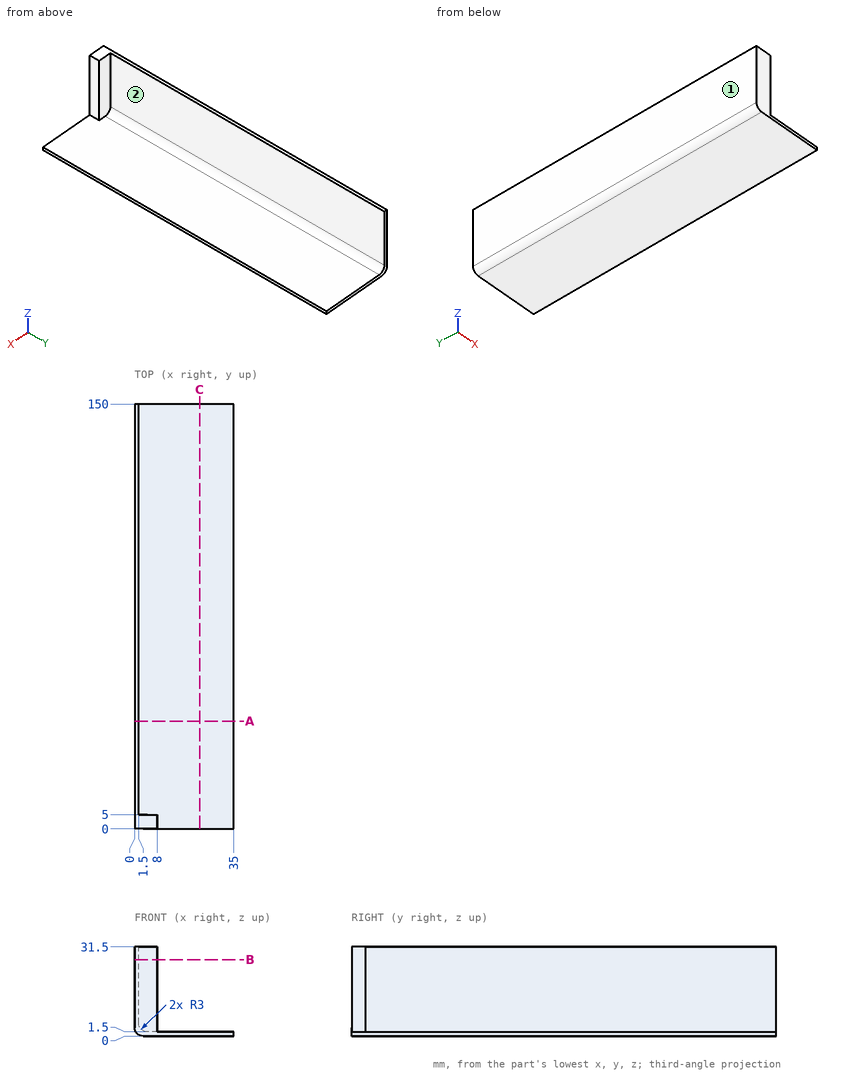
Answer from the drawing. Dimensions are ordinates in mm from the lowest x, y and z of the part. A direction names the side the tool comes from. Coordinates: 2 decimals unless noted, no trailing zeros. Order: outer loops, then holes, each group sorted by start corner. A loop starts at its lowest first (then second) coordinate and runs counter-clockwise, first axis right, second up. Notation, with made-up numbers: M 85,88 L 114,88 A9 ccw 114,99 Z; hole C 62.5,10.5 d6. An arc over 180 degrees is marked long. Put each result on its own line as item: value. Start each with the question number.
Item 1: Given pin 1 Ø8 at (y, z) = (109.5, 19) entering from +X; pin 2 Ø9 at (x, y) = (19.5, 110.5) entering from +Z; pin 3 Ø2.5 at (y, z) = (2, 16.5) entering from +X, each flat-ended and moving along its own axis, determine where each tip first touches the part or whether it passes through.
Item 2: Section B-B, the plane z = 27 is taken. Determine the outline of the cut face in (x, y).
Item 3: For the marked faces 1 and 2, determine the directions among +Z, -Z, +X, -X, +Y, -Y from which every point of the face is accessible in a straight line to the end or side of a thin tool.
Item 4: Section C-C, the plane x = 23 is taken. Determine the outline of the cut face in (y, z), plus the area to 3 significant figures.
Item 5: Section A-A, the plane y = 38 is taken. Determine the outline of the cut face in (x, z).
Item 6: Consider probe 1 along X at (y, z) = (26.5, 30.5); probe 2 along Y at (x, z) = (3, 27.5). Determine where each line is inside the solid, lowest interval first. Write a range as [from, to].
Computed:
1. pin 1: stops at x = 1.5
1. pin 2: stops at z = 1.5
1. pin 3: stops at x = 8
2. outline: M 0,0 L 8,0 L 8,5 L 1.5,5 L 1.5,150 L 0,150 Z
3. face 1: +Z, -Z, -X, +Y, -Y
3. face 2: +Z, +X, +Y
4. outline: M 0,0 L 150,0 L 150,1.5 L 0,1.5 Z
4. area: 225 mm2
5. outline: M 0,3 A3 ccw 3,0 L 35,0 L 35,1.5 L 4.5,1.5 A3 cw 1.5,4.5 L 1.5,31.5 L 0,31.5 Z
6. probe 1: x = [0, 1.5]
6. probe 2: y = [0, 5]
